Input: part model. Units: mm. Frame: model coordinates. A direction names the side the tool comes from. Coordinates: 2 decimals unless noted, no trailing zeros. Loops run counter-clockwise (first coordinate to the right, second up) from the corner with the lowest first, then second, coordinate; pieces in that order, holes last. Notation, with made-up numbers: (12.25, -5.5) - (62.25, -5.5) arc R32 cw to (62.25, 32.5) - close; hole circle Ø3 at (-5, 54.5). An arc over 180 degrees is marked (long way). Answer as CSV lines item,"result". Start each with the question number.
```python
from build123d import *

# Parameters (mm, degrees)
SKETCH1_R           = 2.05
BOSS_EXTRUDE1_DEPTH = 14
SKETCH2_R           = 2.05
CUT_EXTRUDE1_DEPTH  = 28.3


with BuildPart() as part:
    # Sketch1 → Boss-Extrude1 (new body)
    with BuildSketch(Plane(origin=(0, 0, 0), x_dir=(1, 0, 0), z_dir=(0, 1, 0))):
        with BuildLine():
            Line((-19.55, 0), (-19.55, -3.98647317))
            ThreePointArc((-19.55, -3.98647317), (-18.877985148, -6.048632233), (-17.12, -7.318904715))
            ThreePointArc((-17.12, -7.318904715), (0, -10), (17.12, -7.318904715))
            ThreePointArc((17.12, -7.318904715), (18.877985148, -6.048632233), (19.55, -3.98647317))
            Line((19.55, -3.98647317), (19.55, 0))
            ThreePointArc((19.55, 0), (18.22693576, 3.59659757), (14.888553485, 5.478409687))
            Line((14.888553485, 5.478409687), (8.589900273, 6.5))
            ThreePointArc((8.589900273, 6.5), (7.988389953, 6.839065246), (7.75, 7.487100845))
            Line((7.75, 7.487100845), (7.75, 15.9))
            ThreePointArc((7.75, 15.9), (7.603553391, 16.253553391), (7.25, 16.4))
            Line((7.25, 16.4), (0.75, 16.4))
            Line((0.75, 16.4), (0.75, 3.929058411))
            ThreePointArc((0.75, 3.929058411), (0, -4), (-0.75, 3.929058411))
            Line((-0.75, 3.929058411), (-0.75, 16.4))
            Line((-0.75, 16.4), (-7.25, 16.4))
            ThreePointArc((-7.25, 16.4), (-7.603553391, 16.253553391), (-7.75, 15.9))
            Line((-7.75, 15.9), (-7.75, 7.487100845))
            ThreePointArc((-7.75, 7.487100845), (-7.988389953, 6.839065246), (-8.589900273, 6.5))
            Line((-8.589900273, 6.5), (-14.888553485, 5.478409687))
            ThreePointArc((-14.888553485, 5.478409687), (-18.22693576, 3.59659757), (-19.55, 0))
        make_face()
        with Locations((-14, 0)):
            Circle(SKETCH1_R, mode=Mode.SUBTRACT)
        with Locations((14, 0)):
            Circle(SKETCH1_R, mode=Mode.SUBTRACT)
    extrude(amount=BOSS_EXTRUDE1_DEPTH)

    # Sketch2 → Cut-Extrude1 (cut, through all)
    with BuildSketch(Plane(origin=(7.75, 0, 0), x_dir=(0, 0, -1), z_dir=(1, 0, 0))):
        with Locations((11.9, 7)):
            Circle(SKETCH2_R)
    extrude(amount=-CUT_EXTRUDE1_DEPTH, mode=Mode.SUBTRACT)


solid = part.part
```
Item 1: Material intervals for probe 1 along X at (y, z) = (7.25, -9.5); probe 2 along X at (y, z) = (8.25, -1); probe 3 along Y at (x, z) = (4, -11.9), sorted ascending.
Item 2: Contact query for flat-ended pins moving along their axis: P1, Ø2, axis at x = 8.5, y = 4, coming from the -Z side; P2, Ø3, axis at x = 9.5, y = 10.5, coming from the +Z side; P3, Ø6, axis at y = 1.5, z = -1.5, coming from the +X side; P4, Ø8, axis at y = 6.5, z = -7.5, coming from the +X side. Output: stop coordinate, or through.
Item 3: Set-up query: faces 1 (the cylindrical face through (18.86, 6.9, 6.07)), 2 (the flat face through (0.75, 7, -9)), 3 (the flat face through (7.75, 8.5, -9.8)). Return all of +Z, -Z, +X, -X, +Y, -Y with unobstructed straight access to the full face (end or side cutting, diameter ignored); none if empty.
Item 4: Draft query along X for faces 4 (the cylindrical face through (-16.05, 6.9, -0.09)), 5 (the flat face through (11.783, 6.902, -5.982)), 6 (the cylindrical face through (0, 7, 10)), 7 (the flat face through (4, 7, -16.4)). Return one class per face: pulls with the +X half, pulls with the -X half, needs draft (parallel to the pull), parting line crosses it, or undercut.
Item 5: Section query D-D, the plane y = 3.5. Output: boundary loops of the cut face in (x, z), and give its area (3 significant figures).
Item 6: Section query C-C, the plane x = 14. Output: boundary loops of the cut face in (y, z), and give its area (3 significant figures).
Item 7: Section query B-B, the plane z = -11.9. Output: boundary loops of the cut face in (x, y), and give its area (3 significant figures).
Item 8: Section query A-A, the plane y = 7. Give the number of separate pieces and of enclosed holes in the cut face, and give its area (3 significant figures).
Response values:
1,probe 1,"x = -7.75 to -0.75, 0.75 to 7.75"
1,probe 2,"x = -19.46 to -15.79, -12.21 to -3.87, 3.87 to 12.21, 15.79 to 19.46"
1,probe 3,"y = 0 to 4.95, 9.05 to 14"
2,P1,"stops at z = -16.33"
2,P2,"stops at z = 9.43"
2,P3,"stops at x = 19.55"
2,P4,"stops at x = 18.31"
3,face 1,"+Z, +X, +Y, -Y"
3,face 2,"-Z, +Y, -Y"
3,face 3,"-Z, +X, +Y, -Y"
4,face 4,"undercut"
4,face 5,"pulls with the +X half"
4,face 6,"parting line crosses it"
4,face 7,"needs draft"
5,outline,"(-19.55, 0) arc R5.55 ccw to (-14.89, -5.48) - (-8.59, -6.5) arc R1 cw to (-7.75, -7.49) - (-7.75, -15.9) arc R0.5 ccw to (-7.25, -16.4) - (-0.75, -16.4) - (-0.75, -3.93) arc R4 cw (long way) to (0.75, -3.93) - (0.75, -16.4) - (7.25, -16.4) arc R0.5 ccw to (7.75, -15.9) - (7.75, -7.49) arc R1 cw to (8.59, -6.5) - (14.89, -5.48) arc R5.55 ccw to (19.55, 0) - (19.55, 3.99) arc R3.5 ccw to (17.12, 7.32) arc R56 ccw to (-17.12, 7.32) arc R3.5 ccw to (-19.55, 3.99) - close; hole circle Ø4.1 at (-14, 0); hole circle Ø4.1 at (14, 0)"
5,area,"627 mm²"
6,outline,"(0, -5.62) - (14, -5.62) - (14, -2.05) - (0, -2.05) - close; (0, 2.05) - (14, 2.05) - (14, 8.22) - (0, 8.22) - close"
6,area,"136 mm²"
7,outline,"(-7.75, 0) - (-0.75, 0) - (-0.75, 4.95) - (-7.75, 4.95) - close; (-7.75, 9.05) - (-0.75, 9.05) - (-0.75, 14) - (-7.75, 14) - close; (0.75, 0) - (7.75, 0) - (7.75, 4.95) - (0.75, 4.95) - close; (0.75, 9.05) - (7.75, 9.05) - (7.75, 14) - (0.75, 14) - close"
7,area,"139 mm²"
8,separate pieces,"3"
8,enclosed holes,"2"
8,area,"570 mm²"
